Could you check a few things on this model? Use its own coordinates, in mm. Face numbers are marked on the shaded views. Give positions to 0.01 mm unless a question says otherwise; leave off trailing zeros. Write each loop counter-clockwise with the first axis right and the second up, starting at its lowest first coordinate (ties: lowest second). Pieces come first, ordered by that corner, then holes. Notation, with made-up numbers: (45.5, -1.5) - (100.5, -1.5) arc R32 cw to (100.5, 30.5) - close; hole circle Ø7 at (14, -39.5). An arc over 180 degrees is marked (long way). Answer as a JSON object with one key per item and string values. Group by question number.
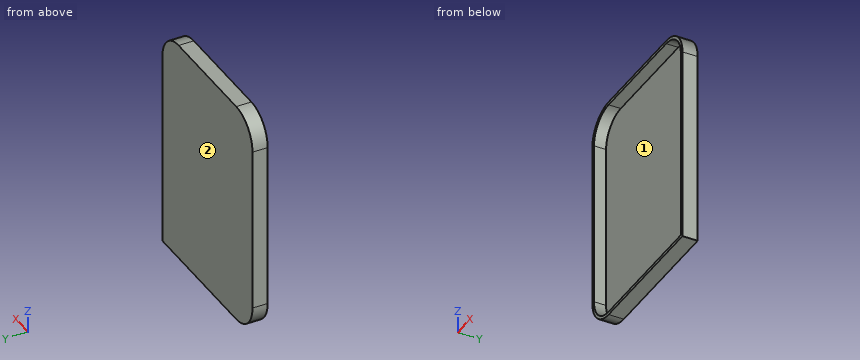
Autodesk Inventor part; units mm, degrees
ref_plane "YZ Plane" through (0, 0, 0) normal (1, 0, 0) x (0, 1, 0)
ref_plane "XZ Plane" through (0, 0, 0) normal (0, 1, 0) x (-1, 0, 0)
ref_plane "XY Plane" through (0, 0, 0) normal (0, 0, 1) x (1, 0, 0)
sketch "Sketch1" plane through (0, 0, 0) normal (0, 1, 0) x (-1, 0, 0)
  line L0 (79.7789, 88.5449) -> (79.7789, -61.4551)
  line L1 (79.7789, -61.4551) -> (-31.0159, -61.4551)
  line L2 (-31.0159, -61.4551) -> (-31.0159, 88.5449)
  line L3 (-31.0159, 88.5449) -> (79.7789, 88.5449)
  point P0 (0, 0)
  dimension "d0" = 150
  dimension "d1" = 110.7948
extrude "Body" add sketch "Sketch1" along normal blind 10
fillet "Fillet6" radius 20 1 edges at (-79.7789, 5, -61.4551)
fillet "Fillet4" radius 20 1 edges at (-79.7789, 5, 88.5449)
fillet "Fillet2" radius 20 1 edges at (31.0159, 5, 88.5449)
shell "Shell2" thickness 2 removed faces 1 at (-42.8473, 0, 31.8782)
properties part number "picaseV2lid"
(1) If we mould it in two halves opening along Z, with no side actions, what happens to the marked faces 1 and 2? For each: +Z half, -Z half, draft (parallel to the pull), parting line (faces both ways), or undercut.
(2) I want a section at B-B, the plane z = 25.5. Please give me the cut outline in (x, y), and give its area (3 significant figures).
(3) Will this pin go through, and if not, where does the flat tip stop? P1, Ø10, axis at x = -23.5, z = -32.5, coming from the -Y side.
(4) I want a section at A-A, the plane y = 3.5. Please give me the cut outline in (x, z), and give its area (3 significant figures).
(5) I need wall thicknesses on L1, parallel to X at y = 3.75, z = 9; L2, parallel to Z at x = -2, y = 3.5; L3, parallel to Y at x = -65, z = 77. Which ranges of each line are inside material? Lowest first, please.
(6) I want a section at C-C, the plane x = 9.5. Please give me the cut outline in (y, z), and give its area (3 significant figures).
Entries:
{
 "1": {"face 1": "undercut", "face 2": "draft"},
 "2": {"outline": "(-79.78, 0) - (-77.78, 0) - (-77.78, 8) - (29.02, 8) - (29.02, 0) - (31.02, 0) - (31.02, 10) - (-79.78, 10) - close", "area": "254 mm^2"},
 "3": {"P1": "y = 8"},
 "4": {"outline": "(-79.78, -41.46) arc R20 ccw to (-59.78, -61.46) - (31.02, -61.46) - (31.02, 68.54) arc R20 ccw to (11.02, 88.54) - (-59.78, 88.54) arc R20 ccw to (-79.78, 68.54) - close; hole (-77.78, -41.46) arc R18 ccw to (-59.78, -59.46) - (29.02, -59.46) - (29.02, 68.54) arc R18 ccw to (11.02, 86.54) - (-59.78, 86.54) arc R18 ccw to (-77.78, 68.54) - close", "area": "978 mm^2"},
 "5": {"L1": "-79.78 to -77.78, 29.02 to 31.02", "L2": "-61.46 to -59.46, 86.54 to 88.54", "L3": "8 to 10"},
 "6": {"outline": "(0, -61.46) - (10, -61.46) - (10, 88.54) - (0, 88.54) - (0, 86.54) - (8, 86.54) - (8, -59.46) - (0, -59.46) - close", "area": "332 mm^2"}
}
